Build history of the part. All positions in model axes, mm. A direction names the side the tool comes from. Round coordinates to 2 decimals unless told otherwise and drop trailing zeros. Write each loop counter-clockwise with the first axis right and the second up, starting at its lowest first coordinate (ties: lowest second). Pieces come first, ordered by that corner, then holes. Notation, with made-up numbers: M 27.25,-38.5 L 45.25,-38.5 A21 cw 45.25,-25.5 Z; hole C 48.25,48.5 d10. An arc over 180 degrees is marked long. Write item = value, one per line. Start each with the question number.
Q1. Pull direction X, two halves, no side cores. Call faces 4 (the flat face through (3.6, 0, 3)), 5 (the flat face through (-3, 0, 4.75)), 6 (the flat face through (-3.6, 0, 3)), 7 (the cylindrical face through (34.3, 0, 3.7)): released by +X, released by -X, zero draft, split by the parting line, or undercut.
Q2. Probe L1, parallel to Y at x = 33.15, z = 6.5; L2, parallel to X at y = -0.5, z = 4.25; L3, parallel to X at y = -0.75, z = 4.5. List the from-to ranges inside material, lowest first.
Q3. Drop flat-ended pins along their axis: P1, Ø1.5, axis at x = 17, z = 0, coming from the +Y side; P2, Ø4.5, axis at x = 18, z = 3.5, coming from the +Y side; P3, Ø2, axis at x = 26, z = 2, coming from the -Y side; P4, Ø1.4, axis at x = -7, y = 0, coming from the +Z side. Give the stop position or say it passes through.
Q4. Band-saw the part on A-A on x = 6.5. Write the cut outline in (y, z), plus the area to 3 significant figures.
Q5. Tool access for faces 1 (the flat face through (0, 0, 7.2)), 2 (the flat face through (2, 0, 2.75)), 3 (the flat face through (11, 0, -1.15)): list every direction of +Z, -Z, +X, -X, +Y, -Y with a clear straight run to the whole face (end or side of a thin tool).
```python
from build123d import *

# Parameters (mm, degrees)
SKETCH_1_W           = 2.4
SKETCH_1_H           = 2.4
EXTRUDE_1_DEPTH      = 7.2
EXTRUDE_2_DEPTH      = 32
EXTRUDE_2_DEPTH_BACK = 12
SKETCH_4_W           = 2.3
SKETCH_4_H           = 2.3
EXTRUDE_3_DEPTH      = 7
EXTRUDE_3_DEPTH_BACK = 2.3
SKETCH_5_R           = 0.35
SKETCH_6_R           = 0.35
CUT_EXTRUDE_1_DEPTH  = 10
FILLET_1_SIZE        = 2.4
FILLET_1_SIZE_2      = 3.2
FILLET_2_R           = 0.5
EXTRUDE_START        = -1.5
SKETCH_7_W           = 1.15
SKETCH_7_H           = 0.5
SKETCH_7_H_2         = 1.3
SKETCH_7_H_3         = 2.3
EXTRUDE_4_DEPTH      = 5.1
SKETCH_8_W           = 7.2
SKETCH_8_H           = 2.3
EXTRUDE_5_DEPTH      = 3.1


with BuildPart() as part:
    # 草图1 → 凸台-拉伸1 (new body)
    with BuildSketch(Plane.XY):
        Rectangle(SKETCH_1_W, SKETCH_1_H)
    extrude(amount=EXTRUDE_1_DEPTH)

    # 草图4 → 凸台-拉伸2 (add, two sides: drawn at the far end of the back side and taken through both)
    with BuildSketch(Plane(origin=(0, 0, 0), x_dir=(0, 0, -1), z_dir=(1, 0, 0)).offset(-EXTRUDE_2_DEPTH_BACK)):
        Rectangle(SKETCH_4_W, SKETCH_4_H)
    extrude(amount=EXTRUDE_2_DEPTH + EXTRUDE_2_DEPTH_BACK)

    # 草图5 → 凸台-拉伸3 (add, two sides: drawn at the far end of the back side and taken through both)
    with BuildSketch(Plane.XY.offset(1.15).offset(-EXTRUDE_3_DEPTH_BACK)):
        with BuildLine():
            Line((32, 0), (32, 1.15))
            Line((32, 1.15), (33.15, 1.15))
            ThreePointArc((33.15, 1.15), (34.3, 0), (33.15, -1.15))
            Line((33.15, -1.15), (32, -1.15))
            Line((32, -1.15), (32, 0))
        make_face()
        with Locations(Location((33.15, 0, 0), (0, 0, 180))):
            Circle(SKETCH_5_R, mode=Mode.SUBTRACT)
    extrude(amount=EXTRUDE_3_DEPTH + EXTRUDE_3_DEPTH_BACK)

    # 草图6 → 切除-拉伸1 (cut)
    with BuildSketch(Plane.ZY.offset(12)):
        Circle(SKETCH_6_R)
    extrude(amount=-CUT_EXTRUDE_1_DEPTH, mode=Mode.SUBTRACT)

    # 圆角1
    # an asymmetric fillet: 3.2, 2.4 mm, written as the material it adds along each edge
    with BuildSketch(Plane(origin=(32, 1.15, 1.15), x_dir=(-1, 0, 0), z_dir=(0, -1, 0))) as fillet_1_piece_1:
        with BuildLine():
            Bezier((FILLET_1_SIZE, 0), (0, 0), (0, -FILLET_1_SIZE_2), weights=[1, 0.707106781, 1])
            Line((0, -FILLET_1_SIZE_2), (0, 0))
            Line((0, 0), (FILLET_1_SIZE, 0))
        make_face()
    extrude(amount=2.3)

    # 圆角2
    fillet_2_edges = [part.edges().sort_by_distance(p)[0] for p in [
        (-6.6, -1.15, 1.15),
        (10.575, -1.15, -1.15),
        (-6.6, 1.15, 1.15),
        (10.575, 1.15, -1.15),
        (34.3, 0, -1.15),
    ]]
    fillet(fillet_2_edges, radius=FILLET_2_R)

    # 草图7 → 凸台-拉伸4 (add)
    with BuildSketch(Plane.XY.offset(1.15).offset(EXTRUDE_START)):
        with Locations((-3.025, 0.9)):
            Rectangle(SKETCH_7_W, SKETCH_7_H)
        with Locations((-3.025, 0)):
            Rectangle(SKETCH_7_W, SKETCH_7_H_2)
        with Locations((-3.025, -0.9)):
            Rectangle(SKETCH_7_W, SKETCH_7_H)
        with Locations((3.025, 0)):
            Rectangle(SKETCH_7_W, SKETCH_7_H_3)
    extrude(amount=EXTRUDE_4_DEPTH)

    # 草图8 → 凸台-拉伸5 (add)
    with BuildSketch(Plane.XY.offset(1.15).offset(EXTRUDE_START)):
        Rectangle(SKETCH_8_W, SKETCH_8_H)
    extrude(amount=EXTRUDE_5_DEPTH)


solid = part.part
```
Conclusion:
q1.face_4 = undercut
q1.face_5 = zero draft
q1.face_6 = released by -X
q1.face_7 = released by +X
q2.L1 = -1.15 to -0.35, 0.35 to 1.15
q2.L2 = -3.6 to -2.45, -1.2 to 1.2, 2.45 to 3.6, 32 to 34.19
q2.L3 = -3.6 to -2.45, -1.2 to 1.2, 2.45 to 3.6, 32 to 34.02
q3.P1 = 1.15
q3.P2 = through
q3.P3 = -1.15
q3.P4 = 1.15
q4.outline = M -1.15,-0.65 A0.5 ccw -0.65,-1.15 L 0.65,-1.15 A0.5 ccw 1.15,-0.65 L 1.15,1.15 L -1.15,1.15 Z
q4.area = 5.18 mm^2
q5.face_1 = +Z, -X, +Y, -Y
q5.face_2 = +Z, +Y, -Y
q5.face_3 = -Z, +X, -X, +Y, -Y
